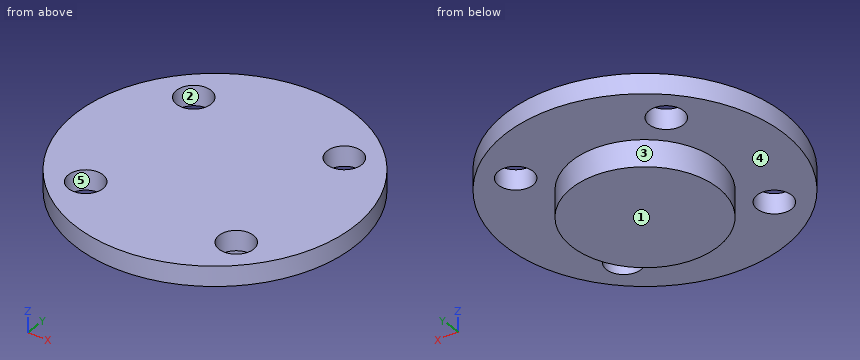
from build123d import *

# Parameters (mm, degrees)
SKETCH_2_R               = 2.6
CUT_EXTRUDE_1_DEPTH      = 3
PATTERN_CIRCULAR_1_COUNT = 4


with BuildPart() as part:
    # Эскиз1 → Повернуть1 (revolve)
    with BuildSketch(Plane(origin=(0, 0, 0), x_dir=(1, 0, 0), z_dir=(0, 1, 0))):
        Polygon((0, 0), (-21, 0), (-21, 3), (-11, 3), (-11, 7), (0, 7), align=None)
    revolve(axis=Axis((0, 0, -7), (0, 0, 1)))

    # Эскиз2 → Вырез-Вытянуть1 (cut)
    with BuildSketch(Plane.XY):
        with Locations((11.313708499, 11.313708499)):
            Circle(SKETCH_2_R)
    cut_extrude_1 = extrude(amount=-CUT_EXTRUDE_1_DEPTH, mode=Mode.SUBTRACT)

    # Круговой массив1: Вырез-Вытянуть1 ×4 about axis
    pattern_circular_1_axis = Axis((0, 0, 0), (0, 0, 1))
    for i in range(1, PATTERN_CIRCULAR_1_COUNT):
        add(cut_extrude_1.rotate(pattern_circular_1_axis, i * 360 / PATTERN_CIRCULAR_1_COUNT), mode=Mode.SUBTRACT)


solid = part.part
Model file for the job. Use its own axes, mm. Face numbers are marked on the shaded views. A direction names the side the tool comes from. Round coordinates to 2 decimals unless told otherwise and drop trailing zeros. Order: outer loops, then holes, each group sorted by start corner. A loop starts at its lowest first (then second) coordinate and runs counter-clockwise, first axis right, second up.
(1) Band-saw the part on B-B (x = 10). List the corners of the cut face in (y, z).
(2) 3-axis set-ups, long thin cutter, end or side, ignore diameter. For the marked faces 4 and 5: which of +Z, -Z, +X, -X, +Y, -Y reach the whole face in a straight line?
(3) Pull direction X, two halves, no side cores. Call the marked faces 1, 2 and 3: released by +X, released by -X, zero draft, split by the parting line, or undercut.
(4) Band-saw the part on C-C (y = 0). List the corners of the cut face in (x, z), then the cut area to 3 significant figures.
(5) Drill centre lines: line 1 (Y direction, x = -10.5, z = -2.5); line 2 (Y direction, x = -11.5, z = -0.25); line 3 (Z direction, x = -8, y = 19). Where is each one in solid material? Low to high.
(6) Pin check, flat tips, straight feed: pin 1 (2 mm diameter, centred on y = 1.5, z = -6, fed in from +X); pin 2 (8.5 mm diameter, centred on x = -11.31, y = 11.31, fed in from -Z); pin 3 (1.5 mm diameter, centred on y = -5, z = -3, fed in from +X). Stop position of each tip, or through.
(7) Band-saw the part on A-A (y = -9.5). List the corners of the cut face in (x, z).
Verdict:
1. outline: (-18.47, -3) - (-13.56, -3) - (-13.56, 0) - (-18.47, 0) - close; (-9.07, -3) - (-4.58, -3) - (-4.58, -7) - (4.58, -7) - (4.58, -3) - (9.07, -3) - (9.07, 0) - (-9.07, 0) - close; (13.56, -3) - (18.47, -3) - (18.47, 0) - (13.56, 0) - close
2. face 4: -Z
2. face 5: +Z, -Z
3. face 1: zero draft
3. face 2: undercut
3. face 3: split by the parting line
4. outline: (-21, -3) - (-11, -3) - (-11, -7) - (11, -7) - (11, -3) - (21, -3) - (21, 0) - (-21, 0) - close
4. area: 214 mm2
5. line 1: y = -18.19 to -13.78, -8.84 to 8.84, 13.78 to 18.19
5. line 2: y = -17.57 to -13.91, -8.72 to 8.72, 13.91 to 17.57
5. line 3: z = -3 to 0
6. pin 1: stops at x = 10.99
6. pin 2: stops at z = -3
6. pin 3: stops at x = 20.57
7. outline: (-18.73, -3) - (-13.18, -3) - (-13.18, 0) - (-18.73, 0) - close; (-9.45, -3) - (-5.55, -3) - (-5.55, -7) - (5.55, -7) - (5.55, -3) - (9.45, -3) - (9.45, 0) - (-9.45, 0) - close; (13.18, -3) - (18.73, -3) - (18.73, 0) - (13.18, 0) - close
